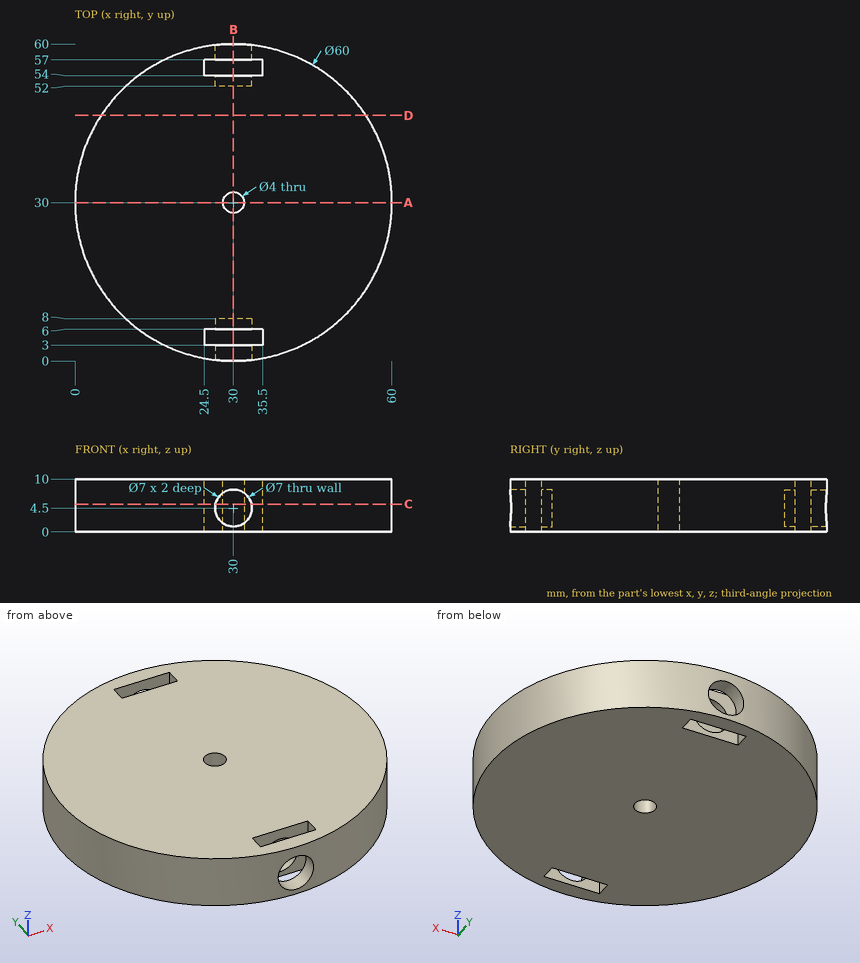
Print and shaded views of the part. All mm, measured from the part's lowest x, y and z. Coordinates: 2 decimals unless noted, no trailing zeros. Order: outer loops, then holes, each group sorted by start corner. A loop starts at its lowest first (then second) coordinate and runs counter-clockwise, first axis right, second up. Notation, with made-up numbers: M 34.25,40.25 L 70.25,40.25 A17 cw 70.25,51.25 Z; hole C 65.5,-8 d10. An arc over 180 degrees is marked long. One line per question, with ' | ' between items. Start each with the question number.
Q1. Flat gauge pins, fed straight in: pin 1 Ø6 at (x, z) = (25, 8) entering from -Y; pin 2 Ø4 at (x, z) = (30, 4.5) entering from +Y; pin 3 Ø2.5 at (y, z) = (56, 4) entering from -X. Where does each tip first touch, or does it go through?
Q2. Saw through at B-B (x = 30). Count the separate pieces of the cut face and the enclosed holes in it, then the cut area to 3 significant figures.
Q3. Probe L1, parallel to Y at x = 33.5, z = 8.25; L2, parallel to Y at x = 26, z = 4.25; L3, parallel to Y at x = 30, z = 4.5. List the from-to ranges inside material, lowest first. Write a range as from..to.
Q4. Saw through at C-C (z = 5.25). List the corners of the cut face in (x, y).
Q5. Saw through at D-D (y = 46.5). List the corners of the cut face in (x, z), then the cut area to 3 significant figures.
Q6. Saw through at A-A (y = 30). List the corners of the cut face in (x, z).
Check values:
1) pin 1: stops at y = 0.07 | pin 2: stops at y = 52 | pin 3: stops at x = 13.05
2) separate pieces: 6 | enclosed holes: 0 | area: 430 mm2
3) L1: y = 0.2..3, 6..54, 57..59.8 | L2: y = 0.27..3, 6..54, 57..59.73 | L3: y = 8..28, 32..52
4) outline: M 24.5,3 L 24.5,6 L 26.58,6 L 26.58,8 L 33.42,8 L 33.42,6 L 35.5,6 L 35.5,3 L 33.42,3 L 33.42,0.2 A30 ccw 33.42,59.8 L 33.42,57 L 35.5,57 L 35.5,54 L 33.42,54 L 33.42,52 L 26.58,52 L 26.58,54 L 24.5,54 L 24.5,57 L 26.58,57 L 26.58,59.8 A30 ccw 26.58,0.2 L 26.58,3 Z; hole C 30,30 d4
5) outline: M 4.95,0 L 55.05,0 L 55.05,10 L 4.95,10 Z | area: 501 mm2
6) outline: M 0,0 L 28,0 L 28,10 L 0,10 Z; M 32,0 L 60,0 L 60,10 L 32,10 Z
